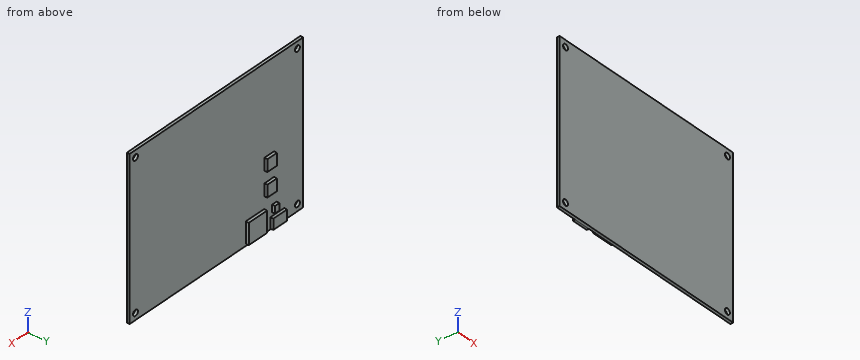
```python
from build123d import *

# Parameters (mm, degrees)
EXTRUDE1_DEPTH        = 1.6002
F_4_CLEARANCE_HOLE1_D = 3.2639
SKETCH5_W             = 6.392759032
SKETCH5_H             = 6.880194124
SKETCH5_W_2           = 9.067841131
SKETCH5_H_2           = 6.084228887
SKETCH5_H_3           = 6.880194125
SKETCH5_W_3           = 12.126342144
SKETCH5_H_4           = 11.868334865
SKETCH5_W_4           = 2.983612243
SKETCH5_H_5           = 4.095154059
BOSS_EXTRUDE1_DEPTH   = 1.5875
BOSS_EXTRUDE1_TAPER   = 3


with BuildPart() as part:
    # Sketch1 → Extrude1 (new body)
    with BuildSketch(Plane(origin=(0, 0, 0), x_dir=(1, 0, 0), z_dir=(0, 1, 0))):
        Polygon((-55.88, -44.45), (49.53, -44.45), (57.15, -44.45), (57.15, -6.35), (57.15, 44.45), (-57.15, 44.45), (-57.15, -6.35), (-57.15, -44.45), align=None)
    extrude(amount=EXTRUDE1_DEPTH)

    # #4 Clearance Hole1 (through all)
    with Locations(Plane(origin=(0, 1.6002, 0), x_dir=(-1, 0, 0), z_dir=(0, 1, 0))):
        with Locations((53.34, -40.64), (-53.34, -40.64), (-53.34, 40.64), (53.34, 40.64)):
            Hole(F_4_CLEARANCE_HOLE1_D / 2)

    # Sketch5 → Boss-Extrude1 (add)
    with BuildSketch(Plane(origin=(0, 1.6002, 0), x_dir=(1, 0, 0), z_dir=(0, 1, 0))):
        with Locations((-34.824290025, 21.681433757)):
            Rectangle(SKETCH5_W, SKETCH5_H)
        with Locations((-40.158796151, 41.104015903)):
            Rectangle(SKETCH5_W_2, SKETCH5_H_2)
        with Locations((-34.824290025, 8.310130462)):
            Rectangle(SKETCH5_W, SKETCH5_H_3)
        with Locations((-25.440323861, 37.525712701)):
            Rectangle(SKETCH5_W_3, SKETCH5_H_4)
        with Locations((-38.228223524, 34.083751803)):
            Rectangle(SKETCH5_W_4, SKETCH5_H_5)
    extrude(amount=BOSS_EXTRUDE1_DEPTH, taper=BOSS_EXTRUDE1_TAPER)


solid = part.part
```
The model under review builds one solid part; all positions refer to its coordinate system, in mm. Coordinates: 2 decimals unless noted, no trailing zeros. Write each loop counter-clockwise with the first axis right and the second up, starting at its lowest first coordinate (ties: lowest second). Pieces come first, ordered by that corner, then holes. Notation, with made-up numbers: (-5, 53) - (14, 53) arc R15 cw to (14, 79) - close; hole circle Ø4 at (75.25, -38.75). An arc over 180 degrees is marked (long way). Write item = value, one per line.
(1) For line 1 (Z direction, x = 53.34, y = 1.05); line 2 (Y direction, x = 40, z = 17); line 3 (X direction, y = 2.35, z = -21), list the stretches that pass through material, from the lowest coordinate up. Write a range as [from, to].
Result sheet:
line_1 = [-44.45, -42.27], [-39.01, 39.01], [42.27, 44.45]
line_2 = [0, 1.6]
line_3 = [-37.98, -31.67]
(2) Consider section D-D, the plane x = -16. Give the boundary of the cut face in (y, z).
Result sheet:
outline = (0, -44.45) - (1.6, -44.45) - (1.6, 44.45) - (0, 44.45) - close
(3) For P1, Ø6, axis at x = -40, z = 4, coming from the +Y side; P2, Ø3, axis at x = -53.34, z = -40.64, coming from the +Y side, all flat-tipped, find the tip position at first contact; note any pin that passes through.
Result sheet:
P1 = 1.6
P2 = through
(4) Consider section C-C, the plane z = -40.64. State how many separate pieces and enclosed holes the cut face has, then the cut area to 3 significant figures.
Result sheet:
separate_pieces = 3
enclosed_holes = 0
area = 206 mm^2
(5) Consider section B-B, the plane z = 40.64. Give the boundary of the cut face in (x, y).
Result sheet:
outline = (-57.15, 0) - (-54.97, 0) - (-54.97, 1.6) - (-57.15, 1.6) - close; (-51.71, 0) - (51.71, 0) - (51.71, 1.6) - (-51.71, 1.6) - close; (54.97, 0) - (57.15, 0) - (57.15, 1.6) - (54.97, 1.6) - close
(6) Consider section A-A, the plane x = -53.34. Give the boundary of the cut face in (y, z), then the cut area to 3 significant figures.
Result sheet:
outline = (0, -44.45) - (1.6, -44.45) - (1.6, -42.27) - (0, -42.27) - close; (0, -39.01) - (1.6, -39.01) - (1.6, 39.01) - (0, 39.01) - close; (0, 42.27) - (1.6, 42.27) - (1.6, 44.45) - (0, 44.45) - close
area = 132 mm^2
